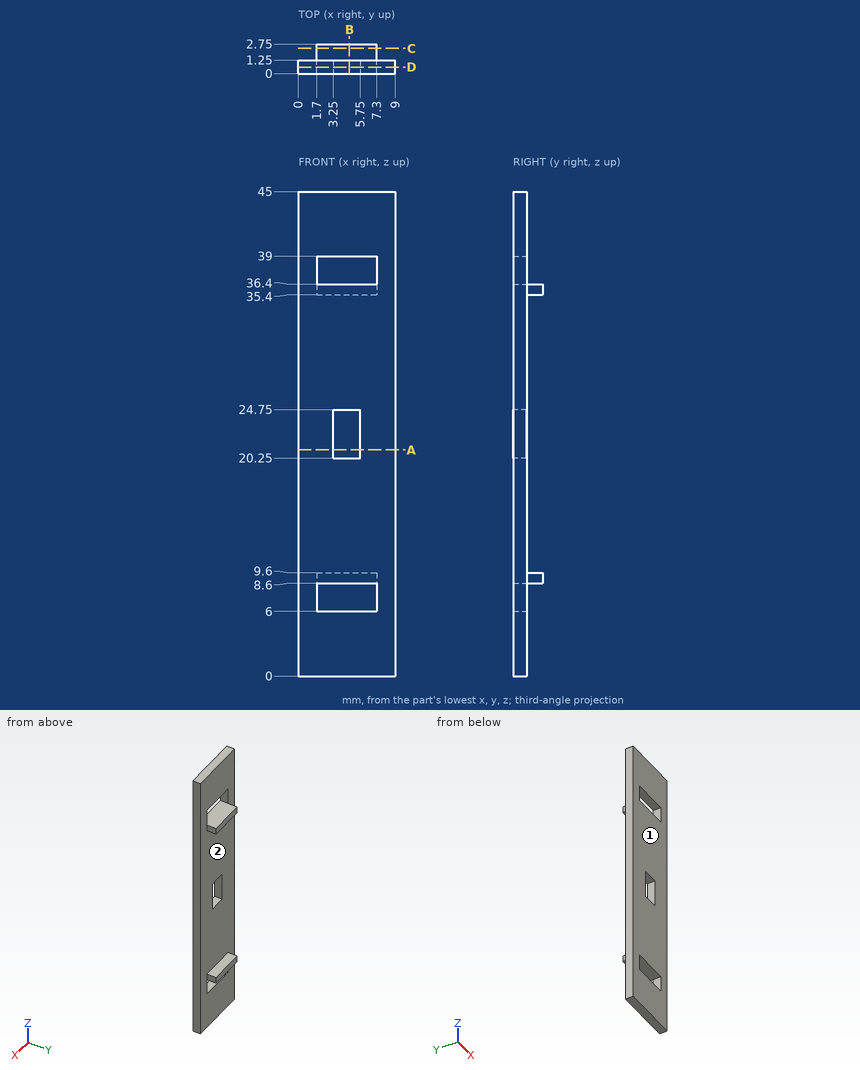
Verification items for this drawing (mm, ordinates from the low corner). Give positions to 0.01 mm unless a question says otherwise; leave off trailing zeros. Write each loop counter-clockwise with the first axis right and the second up, starting at its lowest first coordinate (ties: lowest second). Pieces come first, ordered by that corner, then holes. Notation, with made-up numbers: (-0.5, 41.5) -> (3.5, 41.5) arc R19 cw to (3.5, 52.5) -> close; hole circle Ø4 at (11.25, 86.5). An arc over 180 degrees is marked (long way). Use CSV: the item, a comma, the result in double quotes. Start each with the question number.
Q1. Depth check by flat-ended pin: P1, Ø4, axis at x = 1, z = 18, coming from the +Y side; P2, Ø1.2, axis at x = 5, y = 2, coming from the +Z side; P3, Ø1.4, axis at x = 4, y = 0.5, coming from the -Z side; P4, Ø1.5, axis at x = 6, y = 2.5, coming from the -Z side. Enter the tip coordinate at first touch or a pass-through.
Q2. Cross-section at B-B on x = 4.75. Enter the section's corners in (y, z), and give its area (3 significant figures).
Q3. Cross-section at C-C on y = 2.35. Enter the section's corners in (x, z), and give its area (3 significant figures).
Q4. Cross-section at A-A on z = 21. Enter the section's corners in (x, y).
Q5. Scan lines: line 1 along Z through (x, y) = (3.5, 1.2); line 2 along Z through (x, y) = (7, 0.6); line 3 along Z through (x, y) = (6.25, 1.55). Record each from-to range of solid material in increasing order.
Q6. Release check for a two-part mould opening along Z. For the marked faces 1 and 2 record: +Z half, -Z half, draft (parallel to the pull), parting line (faces both ways), or undercut.
Q7. Cross-section at D-D on y = 0.6. Enter the section's corners in (x, z), and give its area (3 significant figures).
Working result:
1,P1,"stops at y = 1.25"
1,P2,"stops at z = 36.4"
1,P3,"stops at z = 0"
1,P4,"stops at z = 8.6"
2,outline,"(0, 0) -> (1.25, 0) -> (1.25, 6) -> (0, 6) -> close; (0, 8.6) -> (2.75, 8.6) -> (2.75, 9.6) -> (1.25, 9.6) -> (1.25, 20.25) -> (0, 20.25) -> close; (0, 24.75) -> (1.25, 24.75) -> (1.25, 35.4) -> (2.75, 35.4) -> (2.75, 36.4) -> (0, 36.4) -> close; (0, 39) -> (1.25, 39) -> (1.25, 45) -> (0, 45) -> close"
2,area,"47.1 mm^2"
3,outline,"(1.7, 8.6) -> (7.3, 8.6) -> (7.3, 9.6) -> (1.7, 9.6) -> close; (1.7, 35.4) -> (7.3, 35.4) -> (7.3, 36.4) -> (1.7, 36.4) -> close"
3,area,"11.2 mm^2"
4,outline,"(0, 0) -> (3.25, 0) -> (3.25, 1.25) -> (0, 1.25) -> close; (5.75, 0) -> (9, 0) -> (9, 1.25) -> (5.75, 1.25) -> close"
5,line 1,"z = 0 to 6, 8.6 to 20.25, 24.75 to 36.4, 39 to 45"
5,line 2,"z = 0 to 6, 8.6 to 36.4, 39 to 45"
5,line 3,"z = 8.6 to 9.6, 35.4 to 36.4"
6,face 1,"draft"
6,face 2,"undercut"
7,outline,"(0, 0) -> (9, 0) -> (9, 45) -> (0, 45) -> close; hole (1.7, 6) -> (7.3, 6) -> (7.3, 8.6) -> (1.7, 8.6) -> close; hole (1.7, 36.4) -> (7.3, 36.4) -> (7.3, 39) -> (1.7, 39) -> close; hole (3.25, 20.25) -> (5.75, 20.25) -> (5.75, 24.75) -> (3.25, 24.75) -> close"
7,area,"365 mm^2"
